Model file for the job. Use its own axes, mm. A direction names the side the tool comes from. Give positions to 0.01 mm unless a question says otherwise; leave off trailing zeros. Order: outer loops, then holes, each group sorted by start corner. A loop starts at its lowest first (then second) coordinate and runs counter-clockwise, first axis right, second up. Notation, with made-up numbers: (-10, 48) -> (4, 48) arc R19 ccw to (4, 67) -> close; hole circle Ø1 at (88, 56). An arc over 180 degrees is marked (long way). Use CSV: the item, a comma, the result in double quotes. Start each with the question number.
1. Pull direction X, two halves, no side cores. Call faces 1 (the cylindrical face through (0, 45, -22)), 2 (the flat face through (11, 49.5, 11)), 3 (the cylindrical face through (-14.985, 51.965, -0.66)), 4 (the cylindrical face through (-15.413, 44.57, 9.399)): released by +X, released by -X, zero draft, split by the parting line, or undercut.
2. Cut at A-A on x = 0. List the corners of the cut face in (y, z).
3. Cut at D-D on z = 9. List the corners of the cut face in (x, y), then the cut area to 3 significant figures.
4. Cut at C-C on y = 12.5. List the corners of the cut face in (x, z), then the cut area to 3 significant figures.
5. Cut at B-B on z = -20. List the corners of the cut face in (x, y).
6. Wall check: line 1 (X direction, y = 42.25, z = -20); line 2 (X direction, y = 45, z = 10); line 3 (Z direction, x = 0, y = 43). Give the ranges that are in metal, low to high. Write a range as from..to.
7. Drop flat-ended pins along their axis: pin 1 (12 mm diameter, centred on y = 45.5, z = -16, fed in from +X); pin 2 (3 mm diameter, centred on x = 17, z = 11, fed in from +Y); pin 3 (2 mm diameter, centred on x = -17.5, z = 10.5, fed in from +Y); pin 4 (2.5 mm diameter, centred on x = 0, z = -20, fed in from -Y). Give the stop position or say it passes through.
8. 3-axis set-ups, long thin cutter, end or side, ignore diameter. For faces 5 (the flat face through (0, 39.5, -20)), 6 (the cylindrical face through (23.846, 24.404, -7.509)): which of +Z, -Z, +X, -X, +Y, -Y reach the whole face in a straight line?
```python
from build123d import *

# Parameters (mm, degrees)
SKETCH1_R           = 25
BOSS_EXTRUDE1_DEPTH = 49.5
SKETCH2_R           = 15
BOSS_EXTRUDE2_DEPTH = 5
SKETCH3_R           = 4
BOSS_EXTRUDE3_DEPTH = 15
SKETCH4_R           = 2
CUT_EXTRUDE1_DEPTH  = 10


with BuildPart() as part:
    # Sketch1 → Boss-Extrude1 (new body)
    with BuildSketch(Plane(origin=(0, 0, 0), x_dir=(1, 0, 0), z_dir=(0, 1, 0))):
        Circle(SKETCH1_R)
    extrude(amount=BOSS_EXTRUDE1_DEPTH)

    # Sketch2 → Boss-Extrude2 (add)
    with BuildSketch(Plane(origin=(0, 49.5, 0), x_dir=(1, 0, 0), z_dir=(0, 1, 0))):
        Circle(SKETCH2_R)
    extrude(amount=BOSS_EXTRUDE2_DEPTH)

    # Sketch3 → Boss-Extrude3 (add)
    with BuildSketch(Plane(origin=(0, 54.5, 0), x_dir=(1, 0, 0), z_dir=(0, 1, 0))):
        Circle(SKETCH3_R)
    extrude(amount=BOSS_EXTRUDE3_DEPTH)

    # Sketch4 → Cut-Extrude1 (cut)
    with BuildSketch(Plane(origin=(0, 49.5, 0), x_dir=(1, 0, 0), z_dir=(0, 1, 0))):
        with Locations((0, 20)):
            Circle(SKETCH4_R)
        with Locations((17.320508076, -10)):
            Circle(SKETCH4_R)
        with Locations((-17.320508076, -10)):
            Circle(SKETCH4_R)
    extrude(amount=-CUT_EXTRUDE1_DEPTH, mode=Mode.SUBTRACT)


solid = part.part
```
Verdict:
1,face 1,"undercut"
1,face 2,"zero draft"
1,face 3,"split by the parting line"
1,face 4,"undercut"
2,outline,"(0, -25) -> (49.5, -25) -> (49.5, -22) -> (39.5, -22) -> (39.5, -18) -> (49.5, -18) -> (49.5, -15) -> (54.5, -15) -> (54.5, -4) -> (69.5, -4) -> (69.5, 4) -> (54.5, 4) -> (54.5, 15) -> (49.5, 15) -> (49.5, 25) -> (0, 25) -> close"
3,outline,"(-23.32, 0) -> (23.32, 0) -> (23.32, 49.5) -> (19.05, 49.5) -> (19.05, 39.5) -> (15.59, 39.5) -> (15.59, 49.5) -> (12, 49.5) -> (12, 54.5) -> (-12, 54.5) -> (-12, 49.5) -> (-15.59, 49.5) -> (-15.59, 39.5) -> (-19.05, 39.5) -> (-19.05, 49.5) -> (-23.32, 49.5) -> close"
3,area,"2,360 mm^2"
4,outline,"circle Ø50 at (0, 0)"
4,area,"1,960 mm^2"
5,outline,"(-15, 0) -> (15, 0) -> (15, 49.5) -> (2, 49.5) -> (2, 39.5) -> (-2, 39.5) -> (-2, 49.5) -> (-15, 49.5) -> close"
6,line 1,"-15..-2, 2..15"
6,line 2,"-22.91..-19.32, -15.32..15.32, 19.32..22.91"
6,line 3,"-25..-22, -18..25"
7,pin 1,"x = 22.91"
7,pin 2,"y = 49.5"
7,pin 3,"y = 39.5"
7,pin 4,"y = 0"
8,face 5,"+Y"
8,face 6,"+Y, -Y"
